from build123d import *

# Parameters (mm, degrees)
SKETCH_1_W          = 40
SKETCH_1_H          = 95
EXTRUDE_1_DEPTH     = 20
SKETCH_2_R          = 3.15
CUT_EXTRUDE_1_DEPTH = 500
SKETCH_4_W          = 16
SKETCH_4_H          = 24.328759663
CUT_EXTRUDE_2_DEPTH = 500
SKETCH_5_R          = 11.05
CUT_EXTRUDE_3_DEPTH = 20
SKETCH_6_W          = 15.4
SKETCH_6_H          = 15.4
CUT_EXTRUDE_4_DEPTH = 20
SKETCH_7_R          = 1.65
CUT_EXTRUDE_5_DEPTH = 20
SKETCH_8_R          = 1.65
CUT_EXTRUDE_6_DEPTH = 50
FILLET_1_R          = 2


with BuildPart() as part:
    # 草图1 → 凸台-拉伸1 (new body)
    with BuildSketch(Plane.XY):
        with Locations((0, -0.95)):
            Rectangle(SKETCH_1_W, SKETCH_1_H)
    extrude(amount=EXTRUDE_1_DEPTH)

    # 草图2 → 切除-拉伸1 (cut)
    with BuildSketch(Plane(origin=(20, 0, 0), x_dir=(0, 0, -1), z_dir=(1, 0, 0))):
        with Locations((-10, 36.55)):
            Circle(SKETCH_2_R)
    extrude(amount=-CUT_EXTRUDE_1_DEPTH, mode=Mode.SUBTRACT)

    # 草图4 → 切除-拉伸2 (cut)
    with BuildSketch(Plane.XY.offset(20)):
        with Locations((0, 38.714379832)):
            Rectangle(SKETCH_4_W, SKETCH_4_H)
    extrude(amount=-CUT_EXTRUDE_2_DEPTH, mode=Mode.SUBTRACT)

    # 草图5 → 切除-拉伸3 (cut)
    with BuildSketch(Plane.XY.offset(20)):
        with Locations((0, 10.55)):
            Circle(SKETCH_5_R)
    extrude(amount=-CUT_EXTRUDE_3_DEPTH, mode=Mode.SUBTRACT)

    # 草图6 → 切除-拉伸4 (cut)
    with BuildSketch(Plane(origin=(0, 0, 0), x_dir=(-1, 0, 0), z_dir=(0, 0, -1))):
        with Locations((0, -24.95)):
            Rectangle(SKETCH_6_W, SKETCH_6_H)
    extrude(amount=-CUT_EXTRUDE_4_DEPTH, mode=Mode.SUBTRACT)

    # 草图7 → 切除-拉伸5 (cut)
    with BuildSketch(Plane(origin=(0, 0, 0), x_dir=(-1, 0, 0), z_dir=(0, 0, -1))):
        with Locations((4.5, -42.65)):
            Circle(SKETCH_7_R)
        with Locations((-4.5, -42.65)):
            Circle(SKETCH_7_R)
    extrude(amount=-CUT_EXTRUDE_5_DEPTH, mode=Mode.SUBTRACT)

    # 草图8 → 切除-拉伸6 (cut)
    with BuildSketch(Plane(origin=(20, 0, 0), x_dir=(0, 0, -1), z_dir=(1, 0, 0))):
        with Locations((-10, -24.95)):
            Circle(SKETCH_8_R)
    extrude(amount=-CUT_EXTRUDE_6_DEPTH, mode=Mode.SUBTRACT)

    # 圆角1
    fillet_1_edges = [part.edges().sort_by_distance(p)[0] for p in [
        (8, 46.55, 10),
        (-8, 46.55, 10),
        (-8, 26.55, 10),
        (8, 26.55, 10),
        (-20, 46.55, 10),
        (20, 46.55, 10),
    ]]
    fillet(fillet_1_edges, radius=FILLET_1_R)


solid = part.part
The listing builds one solid part. Answer for the finished solid, in the listing's coordinates (mm). A direction names the side the tool comes from. Coordinates: 2 decimals unless noted, no trailing zeros. Write each loop counter-clockwise with the first axis right and the second up, starting at its lowest first coordinate (ties: lowest second). Pieces come first, ordered by that corner, then holes. Notation, with made-up numbers: M -10.5,44 L 1.5,44 A5 ccw 1.5,50 Z; hole C 50.25,72.25 d2. An arc over 180 degrees is marked long. Put each result on its own line as item: value. Start each with the question number.
1. Consider line 1 (Y direction, x = 0, z = 15.5); line 2 (Y direction, x = 12.5, z = 10); line 3 (Y direction, x = -4.5, z = 9.5). Determine where each line is inside the solid, lowest interval first. Write a range as from..to.
2. For a pull along Z with two mould halves and no side action, classify faces 1 (the cylindrical face through (-13.916, 33.475, 10.683)), 2 (the flat face through (-5, 0, 0)), 3 (the flat face through (0, -17.25, 10)) as pulls with the +Z half, pulls with the -Z half, needs draft (parallel to the pull), parting line crosses it, or undercut.
3. A cutting plane is placed at C-C on y = -42.65. Write down the section's boundary in (x, z).
4. A cutting plane is placed at B-B on z = 16.5. Write down the section's boundary in (x, y).
5. A cutting plane is placed at A-A on y = 10.55. Write down the section's boundary in (x, z).
6. A cutting plane is placed at D-D on x = 4.5. Write down the section's boundary in (y, z).
7. Which of the six approach directions +Z, -Z, +X, -X, +Y, -Y give full straight-line access (tool end or side, diameter ignored) to faces 4 (the cylindrical face through (19.43, 45.95, 10.14)), 5 (the flat face through (-8, 33, 10)), 6 (the flat face through (0, -32.65, 10))?
8. Flat-ended cylindrical pins translate along their axes: P1, Ø3.5, axis at x = 1.5, z = 13, coming from the +Y side; P2, Ø3, axis at x = 4.5, y = -42.65, coming from the -Z side. Find the tip coordinate at first contact, or state that the pin passes through.
Resolved:
1. line 1: y = -48.45..-32.65, -17.25..-0.5, 21.6..26.55
1. line 2: y = -48.45..-26.6, -23.3..33.4, 39.7..46.55
1. line 3: y = -48.45..-44.3, -41..-32.65, -17.25..0.46, 20.64..26.55
2. face 1: undercut
2. face 2: pulls with the -Z half
2. face 3: needs draft
3. outline: M -20,0 L -6.15,0 L -6.15,20 L -20,20 Z; M -2.85,0 L 2.85,0 L 2.85,20 L -2.85,20 Z; M 6.15,0 L 20,0 L 20,20 L 6.15,20 Z
4. outline: M -20,-48.45 L 20,-48.45 L 20,44.55 A2 ccw 18,46.55 L 10,46.55 A2 ccw 8,44.55 L 8,28.55 A2 cw 6,26.55 L -6,26.55 A2 cw -8,28.55 L -8,44.55 A2 ccw -10,46.55 L -18,46.55 A2 ccw -20,44.55 Z; hole C 0,10.55 d22.1; hole M -7.7,-32.65 L 7.7,-32.65 L 7.7,-17.25 L -7.7,-17.25 Z; hole C -4.5,-42.65 d3.3; hole C 4.5,-42.65 d3.3
5. outline: M -20,0 L -11.05,0 L -11.05,20 L -20,20 Z; M 11.05,0 L 20,0 L 20,20 L 11.05,20 Z
6. outline: M -48.45,0 L -44.3,0 L -44.3,20 L -48.45,20 Z; M -41,0 L -32.65,0 L -32.65,20 L -41,20 Z; M -17.25,0 L 0.46,0 L 0.46,20 L -17.25,20 Z; M 20.64,0 L 26.55,0 L 26.55,20 L 20.64,20 Z
7. face 4: +Z, -Z, +X, +Y
7. face 5: +Z, -Z, +Y
7. face 6: +Z, -Z
8. P1: stops at y = 26.55
8. P2: passes through
